Autodesk Inventor part; units mm, degrees
ref_plane "YZ Plane" through (0, 0, 0) normal (1, 0, 0) x (0, 1, 0)
ref_plane "XZ Plane" through (0, 0, 0) normal (0, 1, 0) x (-1, 0, 0)
ref_plane "XY Plane" through (0, 0, 0) normal (0, 0, 1) x (1, 0, 0)
sketch "Sketch1" plane through (0, 0, 0) normal (0, 0, 1) x (1, 0, 0)
  line L0 (-47.45, 49.4) -> (47.45, 49.4)
  line L1 (47.45, 49.4) -> (47.45, -49.4)
  line L2 (47.45, -49.4) -> (-47.45, -49.4)
  line L3 (-47.45, -49.4) -> (-47.45, 49.4)
  line L4 (-47.45, 49.4) -> (47.45, -49.4) construction
  line L5 (47.45, 49.4) -> (-47.45, -49.4) construction
  point P0 (0, 0)
  dimension "Comp" = 94.9
  dimension "Larg" = 98.8
extrude "Extrusion1" add sketch "Sketch1" along normal mid plane 6.5
hole "Hole2" at (-33.45, 0, 3.25) direction (0, 0, -1) diameter 13 end through all
hole "Hole3" at (29.25, 0, 3.25) direction (0, 0, -1) diameter 13 end through all
properties part number "Buste3"
Can you work these out from the model? Positions are in its coordinate system, mm. Give positions to 0.01 mm unless a question says otherwise; leave off trailing zeros. Loops run counter-clockwise (first coordinate to the right, second up) from the corner with the lowest first, then second, coordinate; pieces in that order, holes last. Notation, with made-up numbers: M 15.5,3.5 L 31.5,3.5 A22 ccw 31.5,38.5 Z; hole C 81.25,80.5 d11. An arc over 180 degrees is marked long. One line per item, written item: value. Start each with the question number.
1) If we section it at D-D, the plane x = -38: Write out the boundary of the cut face in (y, z), and give its area (3 significant figures).
2) If I drill on line 1 (X direction, y = 0.5, z = 2); line 2 (Y direction, x = 29.25, z = 0.25); line 3 (Y direction, x = 32, z = 0.25), over which ranges is the centre line in solid material (lowest first)? Write a range as [from, to].
3) I'm going to push a flat-ended pin straight in: pin 1 (10.5 mm diameter, centred on x = 29.25, y = 0, fed in from -Z). Where does the tip first touch, or does it pass through?
4) If we section it at B-B, the plane x = 29.25: Write out the boundary of the cut face in (y, z).
5) If we section it at C-C, the plane z = 2: Write out the boundary of the cut face in (x, y).
6) Thinking about a two-plate mould opening in X: for faces 1 (the face through (-39.9, 0.8, 0)), 2 (the face through (-47.45, -1, 0)), 3 (the face through (22.8, 0.8, 0)), 4 (the face through (-1, 49.4, 0)), which applies, +X half, -X half, draft (parallel to the pull), parting line (faces both ways), or undercut?
7) If we section it at A-A, the plane y = 0: Write out the boundary of the cut face in (x, z).
Completed:
1. outline: M -49.4,-3.25 L -4.64,-3.25 L -4.64,3.25 L -49.4,3.25 Z; M 4.64,-3.25 L 49.4,-3.25 L 49.4,3.25 L 4.64,3.25 Z
1. area: 582 mm^2
2. line 1: x = [-47.45, -39.93], [-26.97, 22.77], [35.73, 47.45]
2. line 2: y = [-49.4, -6.5], [6.5, 49.4]
2. line 3: y = [-49.4, -5.89], [5.89, 49.4]
3. pin 1: passes through
4. outline: M -49.4,-3.25 L -6.5,-3.25 L -6.5,3.25 L -49.4,3.25 Z; M 6.5,-3.25 L 49.4,-3.25 L 49.4,3.25 L 6.5,3.25 Z
5. outline: M -47.45,-49.4 L 47.45,-49.4 L 47.45,49.4 L -47.45,49.4 Z; hole C -33.45,0 d13; hole C 29.25,0 d13
6. face 1: undercut
6. face 2: -X half
6. face 3: undercut
6. face 4: draft
7. outline: M -47.45,-3.25 L -39.95,-3.25 L -39.95,3.25 L -47.45,3.25 Z; M -26.95,-3.25 L 22.75,-3.25 L 22.75,3.25 L -26.95,3.25 Z; M 35.75,-3.25 L 47.45,-3.25 L 47.45,3.25 L 35.75,3.25 Z
